from build123d import *

# Parameters (mm, degrees)
SKETCH1_W           = 20
SKETCH1_H           = 3
SKETCH1_W_2         = 3
SKETCH1_H_2         = 20
SKETCH1_R           = 2
SKETCH1_W_3         = 8
SKETCH1_H_3         = 50
BOSS_EXTRUDE1_DEPTH = 3


with BuildPart() as part:
    # Sketch1 → Boss-Extrude1 (new body)
    with BuildSketch(Plane.XY):
        with BuildLine():
            Line((10, -62), (10, -65))
            Line((10, -65), (35, -65))
            Line((35, -65), (35, -63.5))
            ThreePointArc((35, -63.5), (36.65, -61.85), (38.3, -63.5))
            Line((38.3, -63.5), (38.3, -65))
            Line((38.3, -65), (65, -65))
            Line((65, -65), (65, -33.3))
            Line((65, -33.3), (63.5, -33.3))
            ThreePointArc((63.5, -33.3), (61.85, -31.65), (63.5, -30))
            Line((63.5, -30), (65, -30))
            Line((65, -30), (65, -10))
            Line((65, -10), (62, -10))
            Line((62, -10), (62, 10))
            Line((62, 10), (65, 10))
            Line((65, 10), (65, 30))
            Line((65, 30), (63.5, 30))
            ThreePointArc((63.5, 30), (61.85, 31.65), (63.5, 33.3))
            Line((63.5, 33.3), (65, 33.3))
            Line((65, 33.3), (65, 65))
            Line((65, 65), (38.3, 65))
            Line((38.3, 65), (38.3, 63.5))
            ThreePointArc((38.3, 63.5), (36.65, 61.85), (35, 63.5))
            Line((35, 63.5), (35, 65))
            Line((35, 65), (10, 65))
            Line((10, 65), (10, 62))
            Line((10, 62), (-10, 62))
            Line((-10, 62), (-10, 65))
            Line((-10, 65), (-35, 65))
            Line((-35, 65), (-35, 63.5))
            ThreePointArc((-35, 63.5), (-36.65, 61.85), (-38.3, 63.5))
            Line((-38.3, 63.5), (-38.3, 65))
            Line((-38.3, 65), (-65, 65))
            Line((-65, 65), (-65, 33.3))
            Line((-65, 33.3), (-63.5, 33.3))
            ThreePointArc((-63.5, 33.3), (-61.85, 31.65), (-63.5, 30))
            Line((-63.5, 30), (-65, 30))
            Line((-65, 30), (-65, 10))
            Line((-65, 10), (-62, 10))
            Line((-62, 10), (-62, -10))
            Line((-62, -10), (-65, -10))
            Line((-65, -10), (-65, -30))
            Line((-65, -30), (-63.5, -30))
            ThreePointArc((-63.5, -30), (-61.85, -31.65), (-63.5, -33.3))
            Line((-63.5, -33.3), (-65, -33.3))
            Line((-65, -33.3), (-65, -65))
            Line((-65, -65), (-38.3, -65))
            Line((-38.3, -65), (-38.3, -63.5))
            ThreePointArc((-38.3, -63.5), (-36.65, -61.85), (-35, -63.5))
            Line((-35, -63.5), (-35, -65))
            Line((-35, -65), (-10, -65))
            Line((-10, -65), (-10, -62))
            Line((-10, -62), (10, -62))
        make_face()
        with Locations((-40.5, -57.5)):
            Rectangle(SKETCH1_W, SKETCH1_H, mode=Mode.SUBTRACT)
        with Locations((-59.5, -35)):
            Rectangle(SKETCH1_W_2, SKETCH1_H_2, mode=Mode.SUBTRACT)
        with Locations((-5.5, -57.5)):
            Rectangle(SKETCH1_W, SKETCH1_H, mode=Mode.SUBTRACT)
        with Locations((13.5, -35)):
            Rectangle(SKETCH1_W_2, SKETCH1_H_2, mode=Mode.SUBTRACT)
        with Locations((33, -41)):
            Circle(SKETCH1_R, mode=Mode.SUBTRACT)
        with Locations((56, -5)):
            Rectangle(SKETCH1_W_3, SKETCH1_H_3, mode=Mode.SUBTRACT)
        with Locations((-59.5, 0)):
            Rectangle(SKETCH1_W_2, SKETCH1_H_2, mode=Mode.SUBTRACT)
        with Locations((-59.5, 35)):
            Rectangle(SKETCH1_W_2, SKETCH1_H_2, mode=Mode.SUBTRACT)
        with Locations((-40.5, 57.5)):
            Rectangle(SKETCH1_W, SKETCH1_H, mode=Mode.SUBTRACT)
        with Locations((-5.5, 57.5)):
            Rectangle(SKETCH1_W, SKETCH1_H, mode=Mode.SUBTRACT)
        with Locations((13.5, 0)):
            Rectangle(SKETCH1_W_2, SKETCH1_H_2, mode=Mode.SUBTRACT)
        with Locations((33, 8)):
            Circle(SKETCH1_R, mode=Mode.SUBTRACT)
        with BuildLine():
            ThreePointArc((33, 20), (28, 25), (33, 30))
            Line((33, 30), (43, 30))
            ThreePointArc((43, 30), (48, 25), (43, 20))
            Line((43, 20), (33, 20))
        make_face(mode=Mode.SUBTRACT)
        with Locations((13.5, 35)):
            Rectangle(SKETCH1_W_2, SKETCH1_H_2, mode=Mode.SUBTRACT)
        with BuildLine():
            ThreePointArc((43, 50), (48, 45), (43, 40))
            Line((43, 40), (33, 40))
            ThreePointArc((33, 40), (28, 45), (33, 50))
            Line((33, 50), (43, 50))
        make_face(mode=Mode.SUBTRACT)
    extrude(amount=BOSS_EXTRUDE1_DEPTH)


solid = part.part
The model under review builds one solid part; all positions refer to its coordinate system, in mm. A direction names the side the tool comes from. Give positions to 0.01 mm unless a question says otherwise; leave off trailing zeros. Loops run counter-clockwise (first coordinate to the right, second up) from the corner with the lowest first, then second, coordinate; pieces in that order, holes last. Notation, with made-up numbers: (-33, 13.5) -> (15, 13.5) arc R28 ccw to (15, 46.5) -> close; hole circle Ø11 at (40, -8). An arc over 180 degrees is marked (long way). Answer as a JSON object with one key per item and string values. Group by question number.
Q1. Take a section at A-A (y = -2). Write out the cut boundary in (x, z), plus the area to 3 significant figures.
Q2. Take a section at C-C (z = 2.45). State how many separate pieces and enclosed holes the cut face has, plus the area to 3 significant figures.
Q3. Draft analysis for pull direction Y (two halves, no side actions). For faces 1 (the flat face through (15, -35, 1)), 2 (the flat face through (-22, 65, 1)), 3 (the flat face through (-52, -65, 1)), state which applies: pulls with the +Y half, pulls with the -Y half, needs draft (parallel to the pull), parting line crosses it, or undercut.
Q4. Insertion check: pin 1 (0.9 mm diameter, centred on y = -1.5, z = 2, fed in from -X); pin 2 (0.9 mm diameter, centred on x = -37.5, z = 1.5, fed in from +Y). Each pin has a flat end and moves straight along its axis. Give the tip position at first contact, or say it passes through.
Q5. Tool access review of faces 4 (the flat face through (64, -10, 1)), 5 (the flat face through (13, 25, 1)), 6 (the flat face through (65, 20, 1)): name each direction out of +Z, -Z, +X, -X, +Y, -Y from which nothing blocks a thin tool from reaching the whole face with its end or side.
Q6. Wall thickness on line 1 along Y through (x, z) = (33, 1.45); line 2 along Y through (x, z) = (-43.5, 2.8); line 3 along X through (y, z) = (-29, 1.95): over which ranges is each line inside the solid? List them lowest first.
Q7. Take a section at B-B (x = 36.65). Write out the cut boundary in (y, z), plus the area to 3 significant figures.
Answer below:
{
 "1": {"outline": "(-62, 0) -> (-61, 0) -> (-61, 3) -> (-62, 3) -> close; (-58, 0) -> (12, 0) -> (12, 3) -> (-58, 3) -> close; (15, 0) -> (52, 0) -> (52, 3) -> (15, 3) -> close; (60, 0) -> (62, 0) -> (62, 3) -> (60, 3) -> close", "area": "330 mm2"},
 "2": {"separate pieces": "1", "enclosed holes": "15", "area": "15,200 mm2"},
 "3": {"face 1": "undercut", "face 2": "pulls with the +Y half", "face 3": "pulls with the -Y half"},
 "4": {"pin 1": "stops at x = -62", "pin 2": "stops at y = 62.48"},
 "5": {"face 4": "+Z, -Z, +X", "face 5": "+Z, -Z", "face 6": "+Z, -Z, +X, +Y, -Y"},
 "6": {"line 1": "y = -65 to -43, -39 to 6, 10 to 20, 30 to 40, 50 to 65", "line 2": "y = -65 to -59, -56 to 56, 59 to 65", "line 3": "x = -65 to -61, -58 to 12, 15 to 52, 60 to 65"},
 "7": {"outline": "(-61.85, 0) -> (20, 0) -> (20, 3) -> (-61.85, 3) -> close; (30, 0) -> (40, 0) -> (40, 3) -> (30, 3) -> close; (50, 0) -> (61.85, 0) -> (61.85, 3) -> (50, 3) -> close", "area": "311 mm2"}
}
